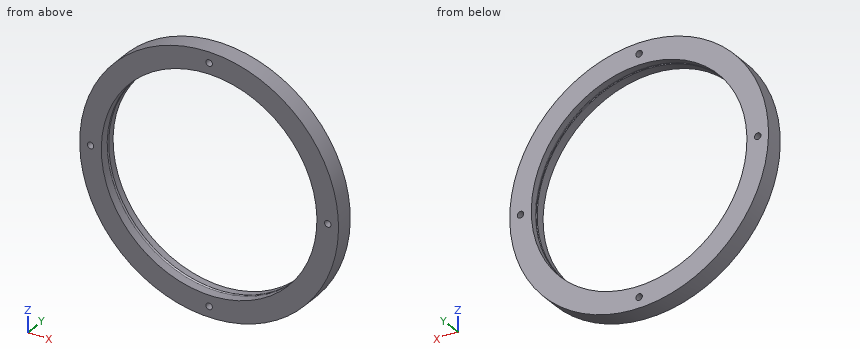
from build123d import *

# Parameters (mm, degrees)
SKETCH_1_R          = 60
SKETCH_1_R_2        = 50
EXTRUDE_2_DEPTH     = 8.4
SKETCH_5_R          = 1.5
CUT_EXTRUDE_1_DEPTH = 10


# Read off the part's stored shape, not the designer's step: the revolve step
with BuildPart() as part:
    # Sketch 1 → Extrude 2 (new body)
    with BuildSketch(Plane(origin=(0, 0, 0), x_dir=(1, 0, 0), z_dir=(0, 1, 0))):
        with Locations(Location((0, 0, 0), (0, 0, 270))):
            Circle(SKETCH_1_R)
        with Locations(Location((0, 0, 0), (0, 0, 270))):
            Circle(SKETCH_1_R_2, mode=Mode.SUBTRACT)
    extrude(amount=EXTRUDE_2_DEPTH)

    # Cut-Revolve 1 outline → Cut-Revolve 1 (revolve, cut)
    with BuildSketch(Plane.XY):
        with BuildLine():
            Line((50, 4.184944399), (50.5, 4.184944399))
            ThreePointArc((50.5, 4.184944399), (50.369306394, 4.797316835), (50, 5.302978388))
            Line((50, 5.302978388), (50, 4.184944399))
        make_face()
    revolve(axis=Axis((0, 0, 0), (0, 1, 0)), mode=Mode.SUBTRACT)

    # Sketch 5 → Cut-Extrude 1 (cut)
    with BuildSketch(Plane(origin=(0, 8.4, 0), x_dir=(1, 0, 0), z_dir=(0, 1, 0))):
        with Locations(Location((0, 55, 0), (0, 0, 270))):
            Circle(SKETCH_5_R)
        with Locations(Location((55, 0, 0), (0, 0, 270))):
            Circle(SKETCH_5_R)
        with Locations(Location((-55, 0, 0), (0, 0, 270))):
            Circle(SKETCH_5_R)
        with Locations(Location((0, -55, 0), (0, 0, 270))):
            Circle(SKETCH_5_R)
    extrude(amount=-CUT_EXTRUDE_1_DEPTH, mode=Mode.SUBTRACT)


solid = part.part
The model under review builds one solid part; all positions refer to its coordinate system, in mm. Round coordinates to 2 decimals unless told otherwise and drop trailing zeros. Order: outer loops, then holes, each group sorted by start corner. A loop starts at its lowest first (then second) coordinate and runs counter-clockwise, first axis right, second up. Notation, with made-up numbers: (28, 7.25) -> (33, 7.25) arc R18 ccw to (33, 33.25) -> close; hole circle Ø3 at (-0.5, -0.75). An arc over 180 degrees is marked (long way). Return JSON: item names as keys, results as strings.
1. Take a section at C-C (x = -55). Write out the cut boundary in (y, z), then the cut area to 3 significant figures.
Answer block:
{"outline": "(0, -23.98) -> (8.4, -23.98) -> (8.4, -1.5) -> (0, -1.5) -> close; (0, 1.5) -> (8.4, 1.5) -> (8.4, 23.98) -> (0, 23.98) -> close", "area": "378 mm²"}
2. Take a section at B-B (y = 2.75). Write out the cut boundary in (x, z).
Answer block:
{"outline": "circle Ø120 at (0, 0); hole circle Ø3 at (-55, 0); hole circle Ø100 at (0, 0); hole circle Ø3 at (0, -55); hole circle Ø3 at (0, 55); hole circle Ø3 at (55, 0)"}
3. For L1, parallel to X at y = 5.75, z = 0; L2, parallel to Y at x = -41.5, z = -28; L3, parallel to Z at x = 38.5, y = 5.25, list the stretches that pass through material, from the lowest coordinate up. Write a range as [from, to].
Answer block:
{"L1": "x = [-60, -56.5], [-53.5, -50], [50, 53.5], [56.5, 60]", "L2": "y = [0, 4.18], [5.24, 8.4]", "L3": "z = [-46.02, -31.99], [31.99, 46.02]"}
4. Take a section at A-A (x = 0). Write out the cut boundary in (y, z), then the cut area to 3 significant figures.
Answer block:
{"outline": "(0, -60) -> (8.4, -60) -> (8.4, -56.5) -> (0, -56.5) -> close; (0, -53.5) -> (8.4, -53.5) -> (8.4, -50) -> (5.3, -50) arc R1.5 cw to (4.18, -50.5) -> (4.18, -50) -> (0, -50) -> close; (0, 50) -> (4.18, 50) -> (4.18, 50.5) arc R1.5 cw to (5.3, 50) -> (8.4, 50) -> (8.4, 53.5) -> (0, 53.5) -> close; (0, 56.5) -> (8.4, 56.5) -> (8.4, 60) -> (0, 60) -> close", "area": "117 mm²"}
5. Insertion check: P1, Ø2, axis at y = 5.5, z = -15.5, coming from the +X side. The pin has a flat end and moves straight along its axis. Give the tip position at first contact, or say it passes through.
Answer block:
{"P1": "stops at x = 58.22"}
